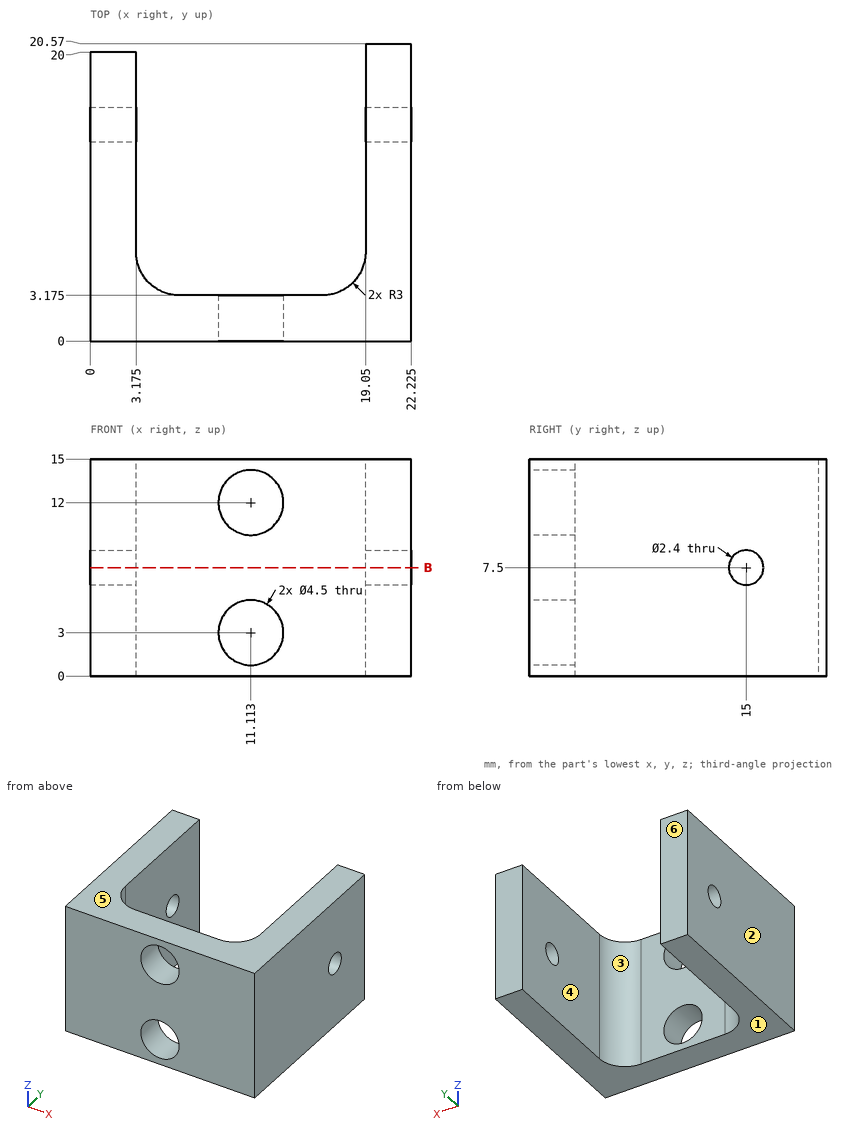
Design review of the part shown in the three views and the two pictorial views. Dimensions are in mm from the part's minimum x, y and z. A direction names the side the tool comes from. Coordinates: 2 decimals unless noted, no trailing zeros. Use one line per item in the form item = value. Start each with the question number.
(1) For probe 1 along Y at (x, z) = (19.8, 7.5); probe 2 along Y at (x, z) = (1.3, 7.5); probe 3 along X at (y, z) = (3, 5) (1 decimal), list the stretches that pass through material, from the lowest coordinate up.
(2) Insertion check: pin 1 (1.4 mm diameter, centred on y = 15, z = 7.5, fed in from +X); pin 2 (1 mm diameter, centred on x = 2, z = 5, fed in from +Y); pin 3 (2 mm diameter, centred on x = 13.5, z = 8.5, fed in from +Y) (1 decimal). Each pin has a flat end and moves straight along its axis. Give the tip position at first contact, or say it passes through.
(3) The part is to be moulded in two halves that separate along X. For the marked faces 1, 2 and 3, say which applies: +X half, -X half, draft (parallel to the pull), parting line (faces both ways), or undercut.
(4) For the marked faces 4, 5 and 6, list the 3-axis set-ups (+Z, -Z, +X, -X, +Y, -Y) from which the entire face can be reached by the end or side of a thin tool; tool diameter is ignored.
(5) Add section B-B on z = 7.5. Give the number of separate pieces and of enclosed holes in the cut face, plus the area to 3 significant figures.
Answer block:
q1.probe_1 = 0 to 13.8, 16.2 to 20.57
q1.probe_2 = 0 to 13.8, 16.2 to 20
q1.probe_3 = 0 to 10.1, 12.1 to 22.2
q2.pin_1 = through
q2.pin_2 = 20
q2.pin_3 = 3.2
q3.face_1 = draft
q3.face_2 = -X half
q3.face_3 = undercut
q4.face_4 = +Z, -Z, +Y
q4.face_5 = +Z, +X, -X, +Y, -Y
q4.face_6 = +Z, -Z, -X, +Y
q5.separate_pieces = 3
q5.enclosed_holes = 0
q5.area = 168 mm²
